Answer from the drawing. Dimensions are ordinates in mm from the lowest x, y and z of the part. A direction names the side the tool comes from. Coordinates: 2 decimals unless noted, no trailing zeros. Order: outer loops, then holes, each group sorted by start corner. A loop starts at its lowest first (then second) coordinate and runs counter-clockwise, first axis right, second up. Notation, with made-up numbers: M -22.5,32.25 L -15.5,32.25 A20 ccw -15.5,63.25 Z; hole C 75,66 d11. An arc over 180 degrees is marked long. Write each question's results on one line, items separated by ' | '.
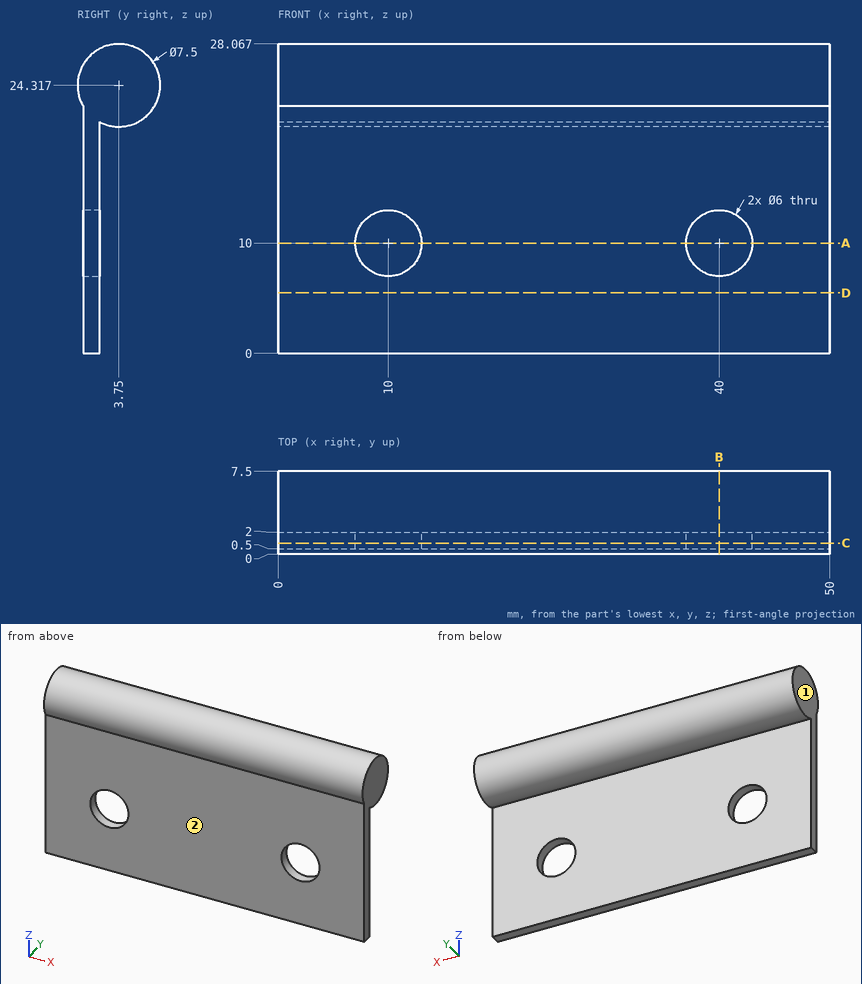
(1) The part is cut by section D-D, the plane z = 5.5. Write down the section's boundary in (x, y).
Conclusion:
outline: M 0,0.5 L 50,0.5 L 50,2 L 0,2 Z
(2) Straight lines are drawn through the part: line 1 (X direction, y = 0.9, z = 10); line 2 (Y direction, x = 8, z = 13); line 3 (Z direction, x = 9, y = 4) (1 decimal). For each, find the intervals that lie inside material, in ascending order.
Conclusion:
line 1: 0 to 7, 13 to 37, 43 to 50 | line 2: 0.5 to 2 | line 3: 20.6 to 28.1
(3) For the marked faces 1 and 2, determine the directions among +Z, -Z, +X, -X, +Y, -Y from which every point of the face is accessible in a straight line to the end or side of a thin tool.
Conclusion:
face 1: +Z, -Z, -X, +Y, -Y | face 2: -Z, +X, -X, -Y
(4) The part is cut by section A-A, the plane z = 10. Write down the section's boundary in (x, y).
Conclusion:
outline: M 0,0.5 L 7,0.5 L 7,2 L 0,2 Z; M 13,0.5 L 37,0.5 L 37,2 L 13,2 Z; M 43,0.5 L 50,0.5 L 50,2 L 43,2 Z
(5) The part is cut by section C-C, the plane y = 1. Write down the section's boundary in (x, z).
Conclusion:
outline: M 0,0 L 50,0 L 50,26.87 L 0,26.87 Z; hole C 10,10 d6; hole C 40,10 d6
(6) The part is cut by section B-B, the plane x = 40. Write down the section's boundary in (y, z).
Conclusion:
outline: M 0.5,0 L 2,0 L 2,7 L 0.5,7 Z; M 0.5,13 L 2,13 L 2,21 A3.75 ccw long 0.5,22.45 Z
(7) Given pin 1 (3 mm diameter, centred on x = 38.5, z = 6, fed in from -Y); pin 2 (6 mm diameter, centred on x = 12, z = 25, fed in from +Y); pin 3 (4 mm diameter, centred on x = 34, z = 11, fed in from +Y); pin 4 (3 mm diameter, centred on x = 32.5, z = 19.5, fed in from +Y), each flat-ended and moving along its own axis, determine where each tip first touches the part or whether it passes through.
Conclusion:
pin 1: y = 0.5 | pin 2: y = 7.5 | pin 3: y = 2 | pin 4: y = 5.5
